Autodesk Inventor part; units mm, degrees
ref_plane "YZ Plane" through (0, 0, 0) normal (1, 0, 0) x (0, 1, 0)
ref_plane "XZ Plane" through (0, 0, 0) normal (0, 1, 0) x (-1, 0, 0)
ref_plane "XY Plane" through (0, 0, 0) normal (0, 0, 1) x (1, 0, 0)
sketch "Sketch1" plane through (0, 0, 0) normal (0, 0, 1) x (1, 0, 0)
  line L0 (-12.7, -12.7) -> (12.7, -12.7)
  line L1 (12.7, -12.7) -> (12.7, 12.7)
  line L2 (12.7, 12.7) -> (-12.7, 12.7)
  line L3 (-12.7, 12.7) -> (-12.7, -12.7)
  line L4 (-12.7, -12.7) -> (12.7, 12.7) construction
  line L5 (12.7, -12.7) -> (-12.7, 12.7) construction
  line L6 (-9.525, -9.525) -> (9.525, -9.525)
  line L7 (9.525, -9.525) -> (9.525, 9.525)
  line L8 (9.525, 9.525) -> (-9.525, 9.525)
  line L9 (-9.525, 9.525) -> (-9.525, -9.525)
  line L10 (-9.525, -9.525) -> (9.525, 9.525) construction
  line L11 (9.525, -9.525) -> (-9.525, 9.525) construction
  point P0 (0, 0)
  dimension "d0" = 25.4
  dimension "d1" = 25.4
  dimension "d2" = 3.175
extrude "Extrusion1" add sketch "Sketch1" along normal blind 879.475
sketch "Sketch2" plane through (12.7, -12.7, 0) normal (1, 0, 0) x (0, 0, -1)
  line L0 (0, 0) -> (0, 25.4)
  line L1 (0, 25.4) -> (-14.6647, 0)
  line L2 (0, 0) -> (-879.475, 0)
  line L3 (0, 0) -> (0, 25.4)
  line L4 (-14.6647, 0) -> (0, 0)
  point P0 (0, 12.7)
  dimension "d10" = 60
extrude "Extrusion2" cut sketch "Sketch2" against normal through all
sketch "Sketch3" plane through (12.7, -12.7, 879.475) normal (1, 0, 0) x (0, 0, -1)
  line L0 (879.475, 25.4) -> (0, 25.4)
  line L1 (0, 25.4) -> (43.9941, 0)
  line L2 (864.8103, 0) -> (0, 0)
  line L3 (0, 0) -> (0, 25.4)
  line L4 (0, 3.175) -> (0, 22.225)
  line L5 (43.9941, 0) -> (0, 0)
  point P0 (879.475, 12.7)
  dimension "d7" = 30
extrude "Extrusion3" cut sketch "Sketch3" against normal through all
properties part number "hypotAluminumExtrusion"
Build history of the part. All positions in model axes, mm. A direction names the side the tool comes from. Round coordinates to 2 decimals unless told otherwise and drop trailing zeros. Loops run counter-clockwise (first coordinate to the right, second up) from the corner with the lowest first, then second, coordinate; pieces in that order, holes last. Notation, with made-up numbers: (-40, 46) -> (-2, 46) arc R14 ccw to (-2, 54) -> close; hole circle Ø8 at (78.25, 84.5). An arc over 180 degrees is marked (long way). One line per item, written item: value. Start each with the question number.
Q1. Probe line 1 along X through (y, z) = (0, 282.5) (3 decimals); line 2 along Y through (x, z) = (-7.5, 842) (3 decimals). List the from-to ranges inside material, lowest first.
Q2. Drop a flat-ended pin along its axis: pin 1 Ø6 at (x, y) = (8.5, -4.5) entering from +Z. Give the stop position or say it passes through.
Q3. Cut at A-A on x = -3.25. List the corners of the cut face in (y, z) (3 decimals), plus the area to 3 significant figures.
Q4. Two-plate mould, pull along X, no slides. Class faces 3 (the face through (0, 9.525, 432)), 4 (the face through (0, 12.7, 434)), 5 (the face through (12.7, 0, 434)): released by +X, released by -X, zero draft, split by the parting line, or undercut.
Q5. 3-axis set-ups, long thin cutter, end or side, ignore diameter. For faces 1 (the face through (0, -9.525, 421)), 2 (the face through (0, -12.7, 419)): which of +Z, -Z, +X, -X, +Y, -Y reach the whole face in a straight line?
Q6. Cut at C-C on y = 5. List the corners of the cut face in (x, z) (3 decimals), plus the area to 3 significant figures.
Q7. Cut at B-B on z = 536. List the corners of the cut face in (x, y) (3 decimals).
Computed:
1. line 1: -12.7 to -9.525, 9.525 to 12.7
1. line 2: 9.525 to 12.7
2. pin 1: z = 854.57
3. outline: (-12.7, 14.665) -> (-9.525, 12.832) -> (-9.525, 840.98) -> (-12.7, 835.481) -> close; (9.525, 1.833) -> (12.7, 0) -> (12.7, 879.475) -> (9.525, 873.976) -> close
3. area: 5,400 mm²
4. face 3: undercut
4. face 4: zero draft
4. face 5: released by +X
5. face 1: +Z, -Z
5. face 2: +Z, -Z, +X, -X, -Y
6. outline: (-12.7, 4.446) -> (-9.525, 4.446) -> (-9.525, 866.138) -> (-12.7, 866.138) -> close; (9.525, 4.446) -> (12.7, 4.446) -> (12.7, 866.138) -> (9.525, 866.138) -> close
6. area: 5,470 mm²
7. outline: (-12.7, -12.7) -> (12.7, -12.7) -> (12.7, 12.7) -> (-12.7, 12.7) -> close; hole (-9.525, -9.525) -> (9.525, -9.525) -> (9.525, 9.525) -> (-9.525, 9.525) -> close
